from build123d import *

# Parameters (mm, degrees)
SKETCH1_W           = 60
SKETCH1_H           = 60
SKETCH1_R           = 3
BOSS_EXTRUDE1_DEPTH = 6
SKETCH2_W           = 60
SKETCH2_H           = 60
SKETCH2_R           = 3
BOSS_EXTRUDE2_DEPTH = 6
BOSS_EXTRUDE3_DEPTH = 3
BOSS_EXTRUDE4_DEPTH = 3


with BuildPart() as part:
    # Sketch1 → Boss-Extrude1 (new body)
    with BuildSketch(Plane.XY):
        with Locations((30, 30)):
            Rectangle(SKETCH1_W, SKETCH1_H)
        with Locations((15, 45)):
            Circle(SKETCH1_R, mode=Mode.SUBTRACT)
        with Locations((15, 15)):
            Circle(SKETCH1_R, mode=Mode.SUBTRACT)
        with BuildLine():
            Line((27.5, 42), (42.5, 42))
            ThreePointArc((42.5, 42), (45.5, 45), (42.5, 48))
            Line((42.5, 48), (27.5, 48))
            ThreePointArc((27.5, 48), (24.5, 45), (27.5, 42))
        make_face(mode=Mode.SUBTRACT)
        with BuildLine():
            Line((27.5, 12), (42.5, 12))
            ThreePointArc((42.5, 12), (45.5, 15), (42.5, 18))
            Line((42.5, 18), (27.5, 18))
            ThreePointArc((27.5, 18), (24.5, 15), (27.5, 12))
        make_face(mode=Mode.SUBTRACT)
    extrude(amount=BOSS_EXTRUDE1_DEPTH)

    # Sketch2 → Boss-Extrude2 (add)
    with BuildSketch(Plane(origin=(60, 0, 0), x_dir=(0, 0, -1), z_dir=(1, 0, 0))):
        with Locations((-30, 30)):
            Rectangle(SKETCH2_W, SKETCH2_H)
        with Locations((-45, 45)):
            Circle(SKETCH2_R, mode=Mode.SUBTRACT)
        with Locations((-45, 15)):
            Circle(SKETCH2_R, mode=Mode.SUBTRACT)
        with BuildLine():
            Line((-32.5, 48), (-17.5, 48))
            ThreePointArc((-17.5, 48), (-14.5, 45), (-17.5, 42))
            Line((-17.5, 42), (-32.5, 42))
            ThreePointArc((-32.5, 42), (-35.5, 45), (-32.5, 48))
        make_face(mode=Mode.SUBTRACT)
        with BuildLine():
            Line((-32.5, 18), (-17.5, 18))
            ThreePointArc((-17.5, 18), (-14.5, 15), (-17.5, 12))
            Line((-17.5, 12), (-32.5, 12))
            ThreePointArc((-32.5, 12), (-35.5, 15), (-32.5, 18))
        make_face(mode=Mode.SUBTRACT)
    extrude(amount=BOSS_EXTRUDE2_DEPTH)

    # Sketch3 → Boss-Extrude3 (add)
    with BuildSketch(Plane(origin=(0, 60, 0), x_dir=(1, 0, 0), z_dir=(0, 1, 0))):
        Polygon((66, 0), (11, 0), (11, -6), (60, -55), (66, -55), align=None)
    extrude(amount=-BOSS_EXTRUDE3_DEPTH)

    # Sketch4 → Boss-Extrude4 (add)
    with BuildSketch(Plane.XZ):
        Polygon((66, 0), (66, 55), (60, 55), (11, 6), (11, 0), align=None)
    extrude(amount=-BOSS_EXTRUDE4_DEPTH)


solid = part.part
Source: CAD feature listing. Evaluate the final solid. Frame: model axes, mm. A direction names the side the tool comes from. Round coordinates to 2 decimals unless told otherwise and drop trailing zeros. Loops run counter-clockwise (first coordinate to the right, second up) from the corner with the lowest first, then second, coordinate; pieces in that order, holes last.
Q1. Ray query, line 1 (Y direction, x = 15, z = 2.15); line 2 (Y direction, x = 36, z = 24); line 3 (X direction, y = 11, z = 22). Return the intervals inside material, ascending.
Q2. Mould query, pull axis X, two halves, no side actions, for faces 5 (the face through (35, 12, 3)), 6 (the face through (47, 60, 17)), 7 (the face through (66, 30, 30)). Classes: pulls with the +X half, pulls with the -X half, needs draft (parallel to the pull), parting line crosses it, or undercut.
Q3. Section B-B, the plane y = 15. Return loops of the section in (x, z), plus the area to 3 significant figures.
Q4. Section D-D, the plane x = 46.5. Return loops of the section in (y, z).
Q5. Section A-A, the plane x = 32.5. Return loops of the section in (y, z).
Q6. First-contact query: P1, Ø5.5, axis at x = 15, y = 45, coming from the +Z side; P2, Ø12, axis at x = 43.5, y = 21, coming from the +Z side; P3, Ø6, axis at y = 16, z = 30.5, coming from the -X side. Flat tips, straight axial feed; report the tip coordinate or a pass-through.
Q7. Section C-C, the plane z = 49.5. Return loops of the section in (x, y).
Q8. Access query for faces 1 (the face through (35, 18, 3)), 2 (the face through (30, 30, 6)), 3 (the face through (47, 0, 17)), 4 (the face through (63, 18, 25)). Directions: +Z, -Z, +X, -X, +Y, -Y. A direction counts if a zero-diameter tool reaches every point of the face in a straight line with its end or side. Return the directions, or none.
Solutions:
1. line 1: y = 0 to 12, 18 to 42, 48 to 60
1. line 2: y = 0 to 3, 57 to 60
1. line 3: x = 60 to 66
2. face 5: undercut
2. face 6: needs draft
2. face 7: pulls with the +X half
3. outline: (0, 0) - (12, 0) - (12, 6) - (0, 6) - close; (18, 0) - (24.5, 0) - (24.5, 6) - (18, 6) - close; (45.5, 0) - (66, 0) - (66, 14.5) - (60, 14.5) - (60, 6) - (45.5, 6) - close; (60, 35.5) - (66, 35.5) - (66, 42) - (60, 42) - close; (60, 48) - (66, 48) - (66, 60) - (60, 60) - close
3. area: 396 mm2
4. outline: (0, 0) - (60, 0) - (60, 41.5) - (57, 41.5) - (57, 6) - (3, 6) - (3, 41.5) - (0, 41.5) - close
5. outline: (0, 0) - (12, 0) - (12, 6) - (3, 6) - (3, 27.5) - (0, 27.5) - close; (18, 0) - (42, 0) - (42, 6) - (18, 6) - close; (48, 0) - (60, 0) - (60, 27.5) - (57, 27.5) - (57, 6) - (48, 6) - close
6. P1: passes through
6. P2: stops at z = 6
6. P3: stops at x = 60
7. outline: (54.5, 0) - (66, 0) - (66, 60) - (54.5, 60) - (54.5, 57) - (60, 57) - (60, 3) - (54.5, 3) - close
8. face 1: +Z, -Z
8. face 2: +Z, -X
8. face 3: +Z, -Z, +X, -X, -Y
8. face 4: +X, -X
